from build123d import *

# Parameters (mm, degrees)
F0_R     = 70
F1_DEPTH = 1


with BuildPart() as f1:
    # F0 (on Top) → F1 (new body)
    with BuildSketch(Plane.XY):
        Circle(F0_R)
        with BuildLine():
            add(Edge.make_bspline(
                [(20.6345475911, -20.9330199765), (20.6345475911, -26.2209165687), (26.2279670975, -26.2209165687)],
                knots=[0, 0, 0, 1, 1, 1], degree=2))
            add(Edge.make_bspline(
                [(26.2279670975, -26.2209165687), (30.9988249119, -26.2209165687), (35.8401880141, -23.776733255)],
                knots=[0, 0, 0, 1, 1, 1], degree=2))
            Line((35.8401880141, -23.776733255), (35.8401880141, -39.7344300823))
            add(Edge.make_bspline(
                [(35.8401880141, -39.7344300823), (28.5076380729, -43.776733255), (17.6263219741, -43.776733255)],
                knots=[0, 0, 0, 1, 1, 1], degree=2))
            add(Edge.make_bspline(
                [(17.6263219741, -43.776733255), (8.0141010576, -43.776733255), (2.8672150411, -39.0646298472)],
                knots=[0, 0, 0, 1, 1, 1], degree=2))
            add(Edge.make_bspline(
                [(2.8672150411, -39.0646298472), (-2.2796709753, -34.3525264395), (-2.2796709753, -25.4688601645)],
                knots=[0, 0, 0, 1, 1, 1], degree=2))
            add(Edge.make_bspline(
                [(-2.2796709753, -25.4688601645), (-2.2796709753, -23.4947121034), (-1.8683901293, -20.9212690952)],
                knots=[0, 0, 0, 1, 1, 1], degree=2))
            add(Edge.make_bspline(
                [(-1.8683901293, -20.9212690952), (-1.4571092832, -18.347826087), (6.9095182139, 22.9917743831)],
                knots=[0, 0, 0, 1, 1, 1], degree=2))
            Line((6.9095182139, 22.9917743831), (-13.2079905993, 22.9917743831))
            Line((-13.2079905993, 22.9917743831), (-27.027027027, -42.2961222092))
            Line((-27.027027027, -42.2961222092), (-49.4947121034, -42.2961222092))
            Line((-49.4947121034, -42.2961222092), (-35.464159812, 22.9917743831))
            Line((-35.464159812, 22.9917743831), (-53.0904817861, 22.9917743831))
            Line((-53.0904817861, 22.9917743831), (-50.9753231492, 33.8025851939))
            Line((-50.9753231492, 33.8025851939), (-36.5687426557, 39.8190364277))
            Line((-36.5687426557, 39.8190364277), (50.2467685076, 39.8190364277))
            Line((50.2467685076, 39.8190364277), (46.7920094007, 22.9917743831))
            Line((46.7920094007, 22.9917743831), (29.1656874266, 22.9917743831))
            Line((29.1656874266, 22.9917743831), (21.2220916569, -16.7262044653))
            add(Edge.make_bspline(
                [(21.2220916569, -16.7262044653), (20.6345475911, -19.6639247944), (20.6345475911, -20.9330199765)],
                knots=[0, 0, 0, 1, 1, 1], degree=2))
        make_face(mode=Mode.SUBTRACT)
    extrude(amount=F1_DEPTH)


solid = f1.part
Model file for the job. Use its own axes, mm. A direction names the side the tool comes from. Coordinates: 2 decimals unless noted, no trailing zeros. Write each loop counter-clockwise with the first axis right and the second up, starting at its lowest first coordinate (ties: lowest second). Pieces come first, ordered by that corner, then holes. Notation, with made-up numbers: (70.25, -34) -> (105.25, -34) arc R9 ccw to (105.25, -25) -> close; hole circle Ø10 at (24.25, -25). An arc over 180 degrees is marked (long way). One line per item, written item: value. Start each with the question number.
1) Which spindle directions (+Z, -Z, +X, -X, +Y, -Y) get a long thin tool onto all of the face, cutting with end or side? Do faces 4 (the face through (-1, 1, 0)), 5 (the face through (-42.578, -10.109, 0.493)). Say none if no direction does.
2) Flat gauge pins, fed straight in: pin 1 Ø0.5 at (x, z) = (5.5, 0.5) entering from -Y; pin 2 Ø0.5 at (y, z) = (-29, 0.5) entering from -X; pin 3 Ø0.5 at (x, z) = (34.5, 0.5) entering from +Y. Where does each tip first touch, or does it go through?
3) Slice it at A-A on x = -47.5. Write the cut outline in (y, z).
4) Slice it at B-B on y = -32.5. Count the separate pieces of the cut face and the enclosed holes in it, then the cut area to 3 significant figures.
5) Probe probe 1 along X at (y, z) = (15, 0.3); probe 2 along X at (y, z) = (-9, 0.65); probe 3 along Y at (x, z) = (15.5, 0.45). List the from-to ranges inside material, lowest first.
6) Pull direction Y, two halves, no side cores. Call faces 1 (the face through (-1, 1, 1)), 2 (the face through (-55.55, -42.594, 0.493)), 3 (the face through (25.25, 3.41, 0.49)): +Y half, -Y half, draft (parallel to the pull), parting line (faces both ways), or undercut.
Answers follow:
1. face 4: -Z, +X, -X, +Y, -Y
1. face 5: +Z, -Z
2. pin 1: y = -69.8
2. pin 2: x = -63.82
2. pin 3: y = 61.05
3. outline: (-51.42, 0) -> (-42.3, 0) -> (-42.3, 1) -> (-51.42, 1) -> close; (-33.01, 0) -> (22.99, 0) -> (22.99, 1) -> (-33.01, 1) -> close; (35.25, 0) -> (51.42, 0) -> (51.42, 1) -> (35.25, 1) -> close
4. separate pieces: 3
4. enclosed holes: 0
4. area: 64.4 mm2
5. probe 1: -68.37 to -37.18, -14.9 to 5.29, 27.57 to 68.37
5. probe 2: -69.42 to -42.34, -19.98 to 0.46, 22.77 to 69.42
5. probe 3: -68.26 to -43.72, 39.82 to 68.26
6. face 1: draft
6. face 2: parting line
6. face 3: undercut
